Study the drawing (mm; zero at the part's minimum x, y, z) and answer. Coordinates: 2 decimals unless noted, no trailing zeros. Loops run counter-clockwise (first coordinate to the right, second up) from the corner with the lowest first, then second, coordinate; pieces in that order, holes last.
Q1. Section B-B (x = 56) is taken. Give the vertices of the cut face in (y, z).
Q2. Straight lines are drawn through the part: line 1 (Y direction, x = 11, z = 0.15); line 2 (X direction, y = 17.5, z = 0.1) (1 decimal); line 3 (Y direction, x = 3.5, z = 1.35). For each, find the intervals that lie inside material, in ascending order.
Q3. Flat-ended cylindrical pins translate along their axes: P1, Ø1.8, axis at x = 4, y = 4, coming from the +Z side; P2, Ø1, axis at y = 38.5, z = 0.5, coming from the -X side. Find the tip coordinate at first contact, or state that the pin passes through.
Q4. Section A-A (y = 19.5) is taken. Give the vertices of the cut face in (x, z) (1 decimal).
Q5. Section D-D (y = 46.5) is taken. Give the vertices of the cut face in (x, z), then the cut area to 3 significant figures.
Q6. Section C-C (z = 1.4) is taken. Count the separate pieces of the cut face and the enclosed holes in it, then the cut area to 3 significant figures.
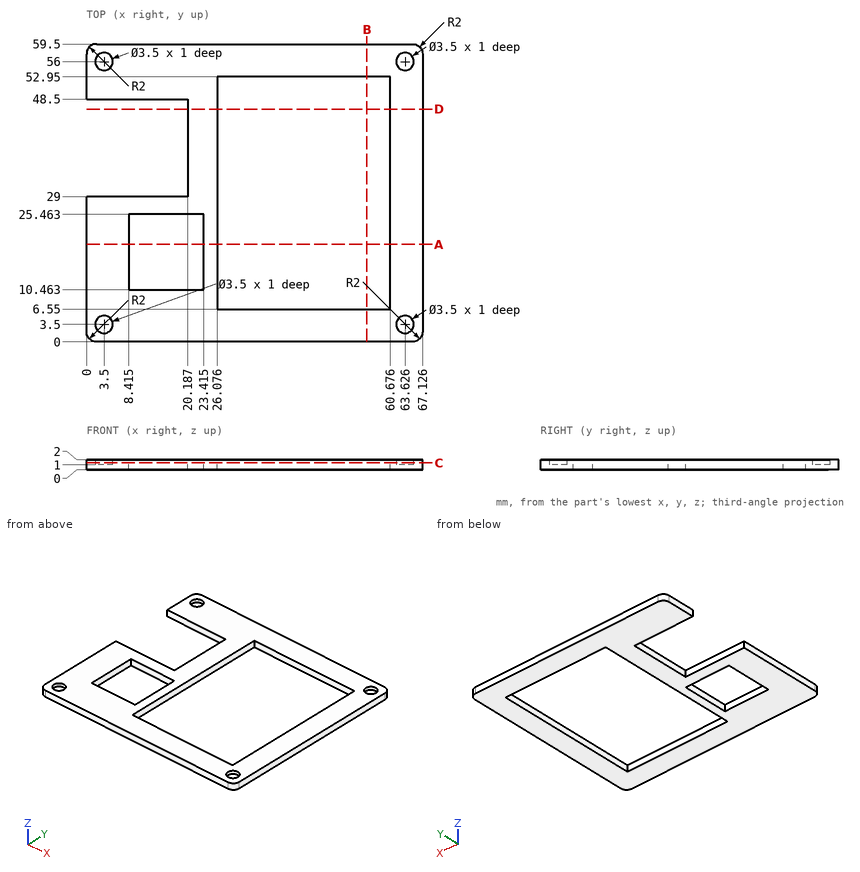
Numbers:
1. outline: (0, 0) - (6.55, 0) - (6.55, 2) - (0, 2) - close; (52.95, 0) - (59.5, 0) - (59.5, 2) - (52.95, 2) - close
2. line 1: y = 0 to 10.46, 25.46 to 29, 48.5 to 59.5
2. line 2: x = 0 to 8.4, 23.4 to 26.1, 60.7 to 67.1
2. line 3: y = 0 to 1.75, 5.25 to 29, 48.5 to 54.25, 57.75 to 59.5
3. P1: stops at z = 1
3. P2: stops at x = 20.19
4. outline: (0, 0) - (8.4, 0) - (8.4, 2) - (0, 2) - close; (23.4, 0) - (26.1, 0) - (26.1, 2) - (23.4, 2) - close; (60.7, 0) - (67.1, 0) - (67.1, 2) - (60.7, 2) - close
5. outline: (20.19, 0) - (26.08, 0) - (26.08, 2) - (20.19, 2) - close; (60.68, 0) - (67.13, 0) - (67.13, 2) - (60.68, 2) - close
5. area: 24.7 mm2
6. separate pieces: 1
6. enclosed holes: 6
6. area: 1,730 mm2
